from build123d import *

# Parameters (mm, degrees)
SKETCH1_W                = 820
SKETCH1_H                = 320
SKETCH1_W_2              = 700
SKETCH1_H_2              = 200
SKETCH1_W_3              = 580
SKETCH1_H_3              = 80
BOSS_EXTRUDE1_DEPTH      = 40
BOSS_EXTRUDE1_DEPTH_BACK = 10
SKETCH1_4_W              = 700
SKETCH1_4_H              = 200
SKETCH1_4_W_2            = 580
SKETCH1_4_H_2            = 80
BOSS_EXTRUDE2_DEPTH      = 40


with BuildPart() as part:
    # Sketch1 → Boss-Extrude1 (new body, two sides)
    with BuildSketch(Plane(origin=(0, 0, 0), x_dir=(1, 0, 0), z_dir=(0, 1, 0))) as boss_extrude1_sk:
        Rectangle(SKETCH1_W, SKETCH1_H)
        Rectangle(SKETCH1_W_2, SKETCH1_H_2, mode=Mode.SUBTRACT)
        Rectangle(SKETCH1_W_2, SKETCH1_H_2)
        Rectangle(SKETCH1_W_3, SKETCH1_H_3, mode=Mode.SUBTRACT)
    extrude(amount=BOSS_EXTRUDE1_DEPTH)
    extrude(boss_extrude1_sk.sketch, amount=-BOSS_EXTRUDE1_DEPTH_BACK)

    # Sketch1_4 → Boss-Extrude2 (add)
    with BuildSketch(Plane(origin=(0, 0, 0), x_dir=(1, 0, 0), z_dir=(0, 1, 0))):
        Rectangle(SKETCH1_4_W, SKETCH1_4_H)
        Rectangle(SKETCH1_4_W_2, SKETCH1_4_H_2, mode=Mode.SUBTRACT)
    extrude(amount=-BOSS_EXTRUDE2_DEPTH)


solid = part.part
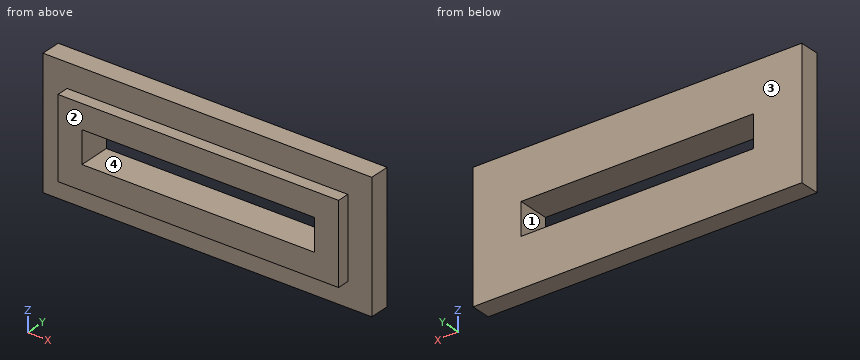
For this review, take the finished solid that the model builds, in its own axes (mm). Face numbers are marked on the shaded views. A direction names the side the tool comes from. Give positions to 0.01 mm unless a question says otherwise; leave off trailing zeros. Loops run counter-clockwise (first coordinate to the right, second up) from the corner with the lowest first, then second, coordinate; pieces in that order, holes last. Notation, with made-up numbers: M 77,70 L 123,70 A26 cw 123,91 Z; hole C 87.25,-1 d9. An arc over 180 degrees is marked long. Answer as a JSON object with one key per item and string values. Group by question number.
Q1. Add section C-C on y = -31. Give the boundary of the cut face in (x, z).
Q2. Add section A-A on x = -46.5. Give the boundary of the cut face in (y, z), and give its area (3 significant figures).
Q3. Add section D-D on z = -90. Give the boundary of the cut face in (x, y).
Q4. Add section B-B on z = -5.5. Give the boundary of the cut face in (x, y).
Q5. Mouldability with a two-part tool opening along X and no side actions: class the marked faces 1 and 2 as +X half, -X half, draft (parallel to the pull), parting line (faces both ways), or undercut.
Q6. For probe 1 along Z at (x, y) = (-82, 23.5); probe 2 along X at (y, z) = (12, -33); probe 3 along Y at (x, z) = (275, 110), list the stretches that pass through material, from the lowest coordinate up. Write a range as [from, to].
Q7. Tool access review of the marked faces 3 and 4: name each direction out of +Z, -Z, +X, -X, +Y, -Y from which nothing blocks a thin tool from reaching the whole face with its end or side.
Q8. Insertion check: P1, Ø24, axis at y = -29, z = 37.5, coming from the +X side; P2, Ø6, axis at x = 211.5, y = -14.5, coming from the +Z side; P3, Ø9, axis at x = -23, y = -23, coming from the -Z side. Each pin has a flat end and moves straight along its axis. Give the tip position at first contact, or say it passes through.
Checked values:
{
 "1": {"outline": "M -350,-100 L 350,-100 L 350,100 L -350,100 Z; hole M -290,-40 L 290,-40 L 290,40 L -290,40 Z"},
 "2": {"outline": "M -40,-100 L -10,-100 L -10,-160 L 40,-160 L 40,-40 L -40,-40 Z; M -40,40 L 40,40 L 40,160 L -10,160 L -10,100 L -40,100 Z", "area": "15,600 mm²"},
 "3": {"outline": "M -410,-10 L -350,-10 L -350,-40 L 350,-40 L 350,-10 L 410,-10 L 410,40 L -410,40 Z"},
 "4": {"outline": "M -410,-10 L -350,-10 L -350,-40 L -290,-40 L -290,40 L -410,40 Z; M 290,-40 L 350,-40 L 350,-10 L 410,-10 L 410,40 L 290,40 Z"},
 "5": {"face 1": "undercut", "face 2": "draft"},
 "6": {"probe 1": "[-160, -40], [40, 160]", "probe 2": "[-410, -290], [290, 410]", "probe 3": "[-10, 40]"},
 "7": {"face 3": "+Z, -Z, +X, -X, +Y", "face 4": "+Y, -Y"},
 "8": {"P1": "x = 350", "P2": "z = 100", "P3": "z = -100"}
}
